For this review, take the finished solid that the model builds, in its own axes (mm). A direction names the side the tool comes from. Give positions to 0.01 mm unless a question says otherwise; leave off trailing zeros. Loops run counter-clockwise (first coordinate to the right, second up) from the corner with the lowest first, then second, coordinate; pieces in that order, holes last. Notation, with made-up numbers: (28, 46) - (47, 46) arc R32 ccw to (47, 81) - close; hole circle Ø10 at (25.5, -0.5). An arc over 180 degrees is marked (long way). Answer as CSV lines item,"result".
from build123d import *

# Parameters (mm, degrees)
F0_R     = 4.95
F1_DEPTH = 4
F2_R     = 2
F3_R     = 2.475
F4_DEPTH = 25
F5_DEPTH = 40


with BuildPart() as f1:
    # F0 (on Top) → F1 (new body)
    with BuildSketch(Plane.XY):
        Circle(F0_R)
    extrude(amount=F1_DEPTH)

    # F2
    f2_edges = [f1.edges().sort_by_distance(p)[0] for p in [
        (-4.95, 0, 4),
    ]]
    fillet(f2_edges, radius=F2_R)

    # F3 (on face) → F4 (join)
    with BuildSketch(Plane(origin=(0, 0, 0), x_dir=(1, 0, 0), z_dir=(0, 0, -1))):
        Circle(F3_R)
    extrude(amount=F4_DEPTH)

    # F3 (on face) → F5 (join)
    with BuildSketch(Plane(origin=(0, 0, 0), x_dir=(1, 0, 0), z_dir=(0, 0, -1))):
        Circle(F3_R)
    extrude(amount=F5_DEPTH)


solid = f1.part
1) Consider section C-C on z = -11. Write out the cut boundary in (x, y) (3 decimals), and give its area (3 significant figures).
From the geometry:
outline,"circle Ø4.95 at (0, 0)"
area,"19.2 mm^2"
2) Wall thickness on line 1 (X direction, y = 0, z = -20) (3 decimals); line 2 (X direction, y = 2.25, z = -38); line 3 (Z direction, x = -3.5, y = -1.5): over which ranges is each line inside the solid? List them lowest first. Write a range as from..to.
From the geometry:
line 1,"x = -2.475..2.475"
line 2,"x = -1.03..1.03"
line 3,"z = 0..3.81"
3) Insertion check: P1, Ø4, axis at x = 0.5, z = -20.5, coming from the -Y side (3 decimals); P2, Ø2, axis at x = -3, y = 3, coming from the -Z side. Each pin has a flat end and moves straight along its axis. Give the tip position at first contact, or say it passes through.
From the geometry:
P1,"stops at y = -2.475"
P2,"stops at z = 0"
4) Machinability: for faces 1 (the flat face through (0, 0, 4)), 2 (the cylindrical face through (2.36, -0.74, -19.72)), which of the approach directions +Z, -Z, +X, -X, +Y, -Y give a long, thin tool a straight path to every point of the face, cutting with its end or side? Answer none if there is none.
From the geometry:
face 1,"+Z, +X, -X, +Y, -Y"
face 2,"-Z"
5) Consider section A-A on y = 0. Write out the cut boundary in (x, z) (3 decimals), and give its area (3 significant figures).
From the geometry:
outline,"(-4.95, 0) - (-2.475, 0) - (-2.475, -40) - (2.475, -40) - (2.475, 0) - (4.95, 0) - (4.95, 2) arc R2 ccw to (2.95, 4) - (-2.95, 4) arc R2 ccw to (-4.95, 2) - close"
area,"236 mm^2"
